Could you check a few things on this model? Use its own coordinates, in mm. A direction names the side the tool comes from. Round coordinates to 2 decimals unless told otherwise and drop trailing zeros. Write each loop counter-clockwise with the first axis right and the second up, starting at its lowest first coordinate (ties: lowest second). Pieces come first, ordered by that corner, then holes. Notation, with made-up numbers: M 3.5,41 L 37.5,41 A19 ccw 37.5,77 Z; hole C -37.75,86 d7. An arc over 180 degrees is marked long. One line per item, written item: value. Start each with the question number.
(1) I want a section at D-D on x = 7. Please give me the cut outline in (y, z).
(2) Thinking about a two-plate mould opening in Y: for faces 1 (the face through (-0.154, -0.175, 8.503)), 2 (the face through (0, 0, 6)), 3 (the face through (-2.05, -15.616, 2.218)), which applies, released by +Y, released by -Y, zero draft, split by the parting line, or undercut?
(3) I want a section at A-A on y = 0. Please give me the cut outline in (x, z).
(4) I want a section at C-C on z = 12. Please give me the cut outline in (x, y), and give its area (3 significant figures).
(5) I want a section at B-B on x = 0. Please give me the cut outline in (y, z).
(6) I'm going to push flat-ended pins straight in: pin 1 Ø1 at (x, y) = (3, 9) entering from -Z; pin 2 Ø4 at (x, y) = (0, 0) entering from -Z; pin 3 Ø5 at (x, z) = (-11, 22) entering from +Y; pin 4 Ø5.5 at (x, z) = (0, 12) entering from +Y. Where does each tip first touch, or does it pass through?
(7) If I drill on L1, parallel to Y at x = 0, z = 29; L2, parallel to Y at x = 0, z = 29.65; L3, parallel to Z at x = 0, y = -4, over which ranges is the centre line in solid material (lowest first)?
(8) Which directions (+Z, -Z, +X, -X, +Y, -Y) give clear straight access to the entire face, cutting with the end or side of a thin tool? Please do faces 4 (the face through (-11.923, 3.755, 0.246)), 5 (the face through (-5, 12, 4.5)), 6 (the face through (-0.1, 10.2, 30)).
Autodesk Inventor part; units mm, degrees
ref_plane "YZ Plane" through (0, 0, 0) normal (1, 0, 0) x (0, 1, 0)
ref_plane "XZ Plane" through (0, 0, 0) normal (0, 1, 0) x (-1, 0, 0)
ref_plane "XY Plane" through (0, 0, 0) normal (0, 0, 1) x (1, 0, 0)
sketch "Sketch1" plane through (0, 0, 0) normal (0, 0, 1) x (1, 0, 0)
  circle A0 centre (0, 0) radius 15.75
  dimension "d0" = 31.5
extrude "Extrusion1" add sketch "Sketch1" along normal blind 4.5
sketch "Sketch2" plane through (0, 0, 4.5) normal (0, 0, 1) x (1, 0, 0)
  circle A0 centre (0, 0) radius 12.5
  dimension "d3" = 25
extrude "Extrusion2" add sketch "Sketch2" along normal blind 25.5
sketch "Sketch3" plane through (0, 0, 30) normal (0, 0, 1) x (1, 0, 0)
  point P0 (0, 0)
  point P1 (0, 0)
hole "Hole1" at (0, 0, 30) direction (0, 0, -1) diameter 5.188 depth 12
sketch "Sketch4" plane through (0, 0, 0) normal (0, 0, -1) x (-1, 0, 0)
  point P0 (0, 0)
  point P1 (0, 0)
hole "Hole2" at (0, 0, 0) direction (0, 0, 1) diameter 5.188 depth 6
sketch "Sketch5" plane through (0, 0, 0) normal (0, 1, 0) x (-1, 0, 0)
  line L0 (15.75, 4.5) -> (-15.75, 4.5)
  point P0 (0, 0)
  point P1 (0, 12)
  dimension "d24" = 12
  dimension "d25" = 7.5
hole "Hole3" at (0, 0, 12) direction (0, -1, 0) diameter 7 end through all both
sketch "Sketch6" plane through (0, 0, 30) normal (0, 0, 1) x (1, 0, 0)
  circle A0 centre (0, 0) radius 10
  dimension "d33" = 20
extrude "Extrusion3" cut sketch "Sketch6" against normal blind 0.5
sketch "Sketch7" plane through (0, 0, 0) normal (0, 0, -1) x (-1, 0, 0)
  circle A0 centre (0, 0) radius 12.5
  dimension "d36" = 25
extrude "Extrusion4" cut sketch "Sketch7" against normal blind 0.5
properties part number "Poste"
Found:
1. outline: M -14.11,0 L -10.36,0 L -10.36,0.5 L 10.36,0.5 L 10.36,0 L 14.11,0 L 14.11,4.5 L 10.36,4.5 L 10.36,30 L 7.14,30 L 7.14,29.5 L -7.14,29.5 L -7.14,30 L -10.36,30 L -10.36,4.5 L -14.11,4.5 Z
2. face 1: zero draft
2. face 2: undercut
2. face 3: split by the parting line
3. outline: M -15.75,0 L -12.5,0 L -12.5,0.5 L -2.59,0.5 L -2.59,6 L 2.59,6 L 2.59,0.5 L 12.5,0.5 L 12.5,0 L 15.75,0 L 15.75,4.5 L 12.5,4.5 L 12.5,30 L 10,30 L 10,29.5 L 2.59,29.5 L 2.59,18 L -2.59,18 L -2.59,29.5 L -10,29.5 L -10,30 L -12.5,30 L -12.5,4.5 L -15.75,4.5 Z; hole C 0,12 d7
4. outline: M -3.5,-12 L -3.5,12 A12.5 ccw Z; M 3.5,-12 A12.5 ccw 3.5,12 Z
4. area: 318 mm²
5. outline: M -15.75,0 L -12.5,0 L -12.5,0.5 L -2.59,0.5 L -2.59,6 L 2.59,6 L 2.59,0.5 L 12.5,0.5 L 12.5,0 L 15.75,0 L 15.75,4.5 L 12.5,4.5 L 12.5,8.5 L -12.5,8.5 L -12.5,4.5 L -15.75,4.5 Z; M -12.5,15.5 L 12.5,15.5 L 12.5,30 L 10,30 L 10,29.5 L 2.59,29.5 L 2.59,18 L -2.59,18 L -2.59,29.5 L -10,29.5 L -10,30 L -12.5,30 Z
6. pin 1: stops at z = 0.5
6. pin 2: stops at z = 6
6. pin 3: stops at y = 9.17
6. pin 4: passes through
7. L1: y = -12.5 to -2.59, 2.59 to 12.5
7. L2: y = -12.5 to -10, 10 to 12.5
7. L3: z = 0.5 to 8.5, 15.5 to 29.5
8. face 4: -Z
8. face 5: +Z
8. face 6: +Z, +X, -X, +Y, -Y
